Design review of the part built by this model. Coordinates are the model's own, in mm. Face numbers are marked on the shaded views. Coordinates: 2 decimals unless noted, no trailing zeros. Loops run counter-clockwise (first coordinate to the right, second up) from the corner with the lowest first, then second, coordinate; pieces in that order, holes last. Notation, with made-up numbers: (52, 44) - (75, 44) arc R24 cw to (75, 61) - close; hole circle Ø3 at (58.5, 49.5). An arc over 180 degrees is marked (long way). Answer in a Markdown table with one row per item. Add a question column.
(1) The part is to be moulded in two halves that separate along Y. For the marked faces 1 and 2, say which applies: released by +Y, released by -Y, zero draft, split by the parting line, or undercut.
(2) We need section A-A, the plane y = 1.5. Give the number of separate pieces and of enclosed holes in the cut face, plus the area to 3 significant figures.
(3) Clearance check with flat-ended pins moving along their axes: pin 1 (0.8 mm diameter, centred on x = 73, z = -5.5, fed in from +Y); pin 2 (0.8 mm diameter, centred on y = 1.5, z = -10.5, fed in from -X). State where each tip first meets the part, or that it passes through.
(4) We need section B-B, the plane x = 31. Write out the cut boundary in (y, z), plus the area to 3 significant figures.
(5) To check wall thickness, follow L1, parallel to X at y = 0.85, z = -2.25; L2, parallel to Y at x = 48, z = -1; L3, parallel to Z at x = 91, y = 0.95. State the ranges of each line that lie inside material, in increasing order. Write a range as [from, to].
from build123d import *

# Parameters (mm, degrees)
BOSS_EXTRUDE1_DEPTH = 2
SKETCH2_W           = 1
SKETCH2_H           = 20
CUT_EXTRUDE1_DEPTH  = 1


with BuildPart() as part:
    # Sketch1 → Boss-Extrude1 (new body)
    with BuildSketch(Plane(origin=(0, 0, 0), x_dir=(1, 0, 0), z_dir=(0, 1, 0))):
        Polygon((122.5, 2.5), (122.5, 0), (150, 0), (150, 20), (122.5, 20), (122.5, 17.5), (117.5, 17.5), (117.5, 20), (92.5, 20), (92.5, 17.5), (87.5, 17.5), (87.5, 20), (62.5, 20), (62.5, 17.5), (57.5, 17.5), (57.5, 20), (32.5, 20), (32.5, 17.5), (27.5, 17.5), (27.5, 20), (0, 20), (0, 0), (27.5, 0), (27.5, 2.5), (32.5, 2.5), (32.5, 0), (57.5, 0), (57.5, 2.5), (62.5, 2.5), (62.5, 0), (87.5, 0), (87.5, 2.5), (92.5, 2.5), (92.5, 0), (117.5, 0), (117.5, 2.5), align=None)
    extrude(amount=BOSS_EXTRUDE1_DEPTH)

    # Sketch2 → Cut-Extrude1 (cut)
    with BuildSketch(Plane(origin=(0, 2, 0), x_dir=(1, 0, 0), z_dir=(0, 1, 0))):
        with Locations((3, 10)):
            Rectangle(SKETCH2_W, SKETCH2_H)
        with Locations((8, 10)):
            Rectangle(SKETCH2_W, SKETCH2_H)
        with Locations((13, 10)):
            Rectangle(SKETCH2_W, SKETCH2_H)
        with Locations((18, 10)):
            Rectangle(SKETCH2_W, SKETCH2_H)
        with Locations((23, 10)):
            Rectangle(SKETCH2_W, SKETCH2_H)
        with Locations((38, 10)):
            Rectangle(SKETCH2_W, SKETCH2_H)
        with Locations((43, 10)):
            Rectangle(SKETCH2_W, SKETCH2_H)
        with Locations((48, 10)):
            Rectangle(SKETCH2_W, SKETCH2_H)
        with Locations((53, 10)):
            Rectangle(SKETCH2_W, SKETCH2_H)
        with Locations((68, 10)):
            Rectangle(SKETCH2_W, SKETCH2_H)
        with Locations((73, 10)):
            Rectangle(SKETCH2_W, SKETCH2_H)
        with Locations((78, 10)):
            Rectangle(SKETCH2_W, SKETCH2_H)
        with Locations((83, 10)):
            Rectangle(SKETCH2_W, SKETCH2_H)
        with Locations((98, 10)):
            Rectangle(SKETCH2_W, SKETCH2_H)
        with Locations((103, 10)):
            Rectangle(SKETCH2_W, SKETCH2_H)
        with Locations((108, 10)):
            Rectangle(SKETCH2_W, SKETCH2_H)
        with Locations((113, 10)):
            Rectangle(SKETCH2_W, SKETCH2_H)
        with Locations((128, 10)):
            Rectangle(SKETCH2_W, SKETCH2_H)
        with Locations((133, 10)):
            Rectangle(SKETCH2_W, SKETCH2_H)
        with Locations((138, 10)):
            Rectangle(SKETCH2_W, SKETCH2_H)
        with Locations((143, 10)):
            Rectangle(SKETCH2_W, SKETCH2_H)
        with Locations((148, 10)):
            Rectangle(SKETCH2_W, SKETCH2_H)
    extrude(amount=-CUT_EXTRUDE1_DEPTH, mode=Mode.SUBTRACT)


solid = part.part
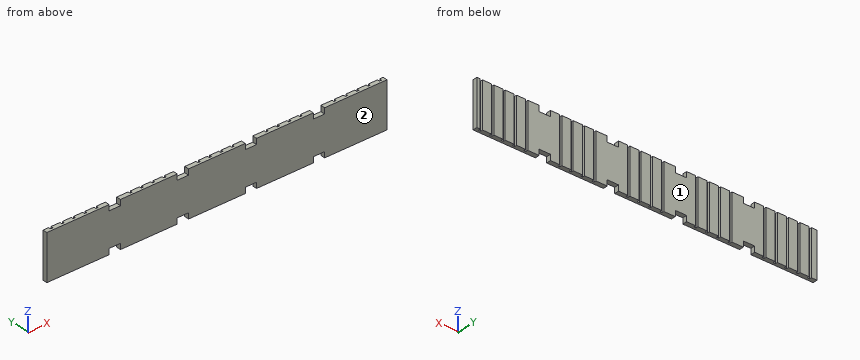
Responses:
| question | item | result |
|---|---|---|
| 1 | face 1 | released by +Y |
| 1 | face 2 | released by -Y |
| 2 | separate pieces | 23 |
| 2 | enclosed holes | 0 |
| 2 | area | 2,460 mm2 |
| 3 | pin 1 | stops at y = 1 |
| 3 | pin 2 | stops at x = 0 |
| 4 | outline | (0, -17.5) - (2, -17.5) - (2, -2.5) - (0, -2.5) - close |
| 4 | area | 30.0 mm2 |
| 5 | L1 | x = [0, 27.5], [32.5, 57.5], [62.5, 87.5], [92.5, 117.5], [122.5, 150] |
| 5 | L2 | y = [0, 1] |
| 5 | L3 | z = [-17.5, -2.5] |
